from build123d import *

# Parameters (mm, degrees)
F0_W       = 52.5
F0_H       = 3
F1_DEPTH   = 6
F0_H_2     = 6
F2_DEPTH   = 3
F4_SIZE    = 2.99999
F5_SIZE2   = 6
F5_SIZE    = 12
F5_2_SIZE2 = 6
F5_2_SIZE  = 12
F6_W       = 4
F6_H       = 39
F7_DEPTH   = 2
F8_SIZE    = 1.99999
F10_DEPTH  = 3
F13_DEPTH  = 3
F12_W      = 4
F12_H      = 39
F15_DEPTH  = 2
F16_SIZE   = 1.99999
F17_SIZE   = 1.99999
F18_DEPTH  = 25
F19_R      = 5


# Not quite as in the source:
# - a fillet or chamfer is up to 0.001 mm smaller than in the source, because OpenCascade refuses the exact size


with BuildPart() as f1:
    # F0 (on Top) → F1 (new body)
    with BuildSketch(Plane.XY):
        with Locations((0, 27)):
            Rectangle(F0_W, F0_H)
        with Locations((0, 24)):
            Rectangle(F0_W, F0_H)
    extrude(amount=F1_DEPTH)


with BuildPart() as f1b:
    # F0 (on Top) → F1, piece 2 (new body)
    with BuildSketch(Plane.XY):
        Rectangle(F0_W, F0_H_2)
    extrude(amount=F1_DEPTH)


with BuildPart() as f1c:
    # F0 (on Top) → F1, piece 3 (new body)
    with BuildSketch(Plane.XY):
        with Locations((0, -24)):
            Rectangle(F0_W, F0_H)
        with Locations((0, -27)):
            Rectangle(F0_W, F0_H)
    extrude(amount=F1_DEPTH)


with BuildPart() as f2:
    # F0 (on Top) → F2 (new body)
    with BuildSketch(Plane.XY):
        Polygon((-38.25, 28.5), (-38.25, -28.5), (-38.25, -31.5), (-35.25, -31.5), (35.25, -31.5), (38.25, -31.5), (38.25, -28.5), (38.25, 28.5), (38.25, 31.5), (35.25, 31.5), (-35.25, 31.5), (-38.25, 31.5), align=None)
        with BuildLine():
            Line((-26.25, -25.5), (-29.75, -25.5))
            ThreePointArc((-29.75, -25.5), (-34.017766953, -27.267766953), (-32.25, -23))
            Line((-32.25, -23), (-32.25, -2.5))
            ThreePointArc((-32.25, -2.5), (-34.75, 0), (-32.25, 2.5))
            Line((-32.25, 2.5), (-32.25, 23))
            ThreePointArc((-32.25, 23), (-34.017766953, 27.267766953), (-29.75, 25.5))
            Line((-29.75, 25.5), (-26.25, 25.5))
            Line((-26.25, 25.5), (-26.25, 28.5))
            Line((-26.25, 28.5), (26.25, 28.5))
            Line((26.25, 28.5), (26.25, 25.5))
            Line((26.25, 25.5), (29.75, 25.5))
            ThreePointArc((29.75, 25.5), (32.25, 28), (34.75, 25.5))
            ThreePointArc((34.75, 25.5), (34.017766953, 23.732233047), (32.25, 23))
            Line((32.25, 23), (32.25, 2.5))
            ThreePointArc((32.25, 2.5), (34.017766953, 1.767766953), (34.75, 0))
            ThreePointArc((34.75, 0), (34.017766953, -1.767766953), (32.25, -2.5))
            Line((32.25, -2.5), (32.25, -23))
            ThreePointArc((32.25, -23), (34.017766953, -23.732233047), (34.75, -25.5))
            ThreePointArc((34.75, -25.5), (32.25, -28), (29.75, -25.5))
            Line((29.75, -25.5), (26.25, -25.5))
            Line((26.25, -25.5), (26.25, -28.5))
            Line((26.25, -28.5), (-26.25, -28.5))
            Line((-26.25, -28.5), (-26.25, -25.5))
        make_face(mode=Mode.SUBTRACT)
        with BuildLine():
            ThreePointArc((-32.25, -23), (-30.482233047, -23.732233047), (-29.75, -25.5))
            Line((-29.75, -25.5), (-26.25, -25.5))
            Line((-26.25, -25.5), (-26.25, -22.5))
            Line((-26.25, -22.5), (26.25, -22.5))
            Line((26.25, -22.5), (26.25, -25.5))
            Line((26.25, -25.5), (29.75, -25.5))
            ThreePointArc((29.75, -25.5), (30.482233047, -23.732233047), (32.25, -23))
            Line((32.25, -23), (32.25, -2.5))
            ThreePointArc((32.25, -2.5), (29.75, 0), (32.25, 2.5))
            Line((32.25, 2.5), (32.25, 23))
            ThreePointArc((32.25, 23), (30.482233047, 23.732233047), (29.75, 25.5))
            Line((29.75, 25.5), (26.25, 25.5))
            Line((26.25, 25.5), (26.25, 22.5))
            Line((26.25, 22.5), (-26.25, 22.5))
            Line((-26.25, 22.5), (-26.25, 25.5))
            Line((-26.25, 25.5), (-29.75, 25.5))
            ThreePointArc((-29.75, 25.5), (-30.482233047, 23.732233047), (-32.25, 23))
            Line((-32.25, 23), (-32.25, 2.5))
            ThreePointArc((-32.25, 2.5), (-30.482233047, 1.767766953), (-29.75, 0))
            ThreePointArc((-29.75, 0), (-30.482233047, -1.767766953), (-32.25, -2.5))
            Line((-32.25, -2.5), (-32.25, -23))
        make_face()
        with BuildLine():
            ThreePointArc((-23.25, -19.5), (-25.3713203436, -18.6213203436), (-26.25, -16.5))
            Line((-26.25, -16.5), (-26.25, -9))
            ThreePointArc((-26.25, -9), (-25.3713203436, -6.8786796564), (-23.25, -6))
            Line((-23.25, -6), (23.25, -6))
            ThreePointArc((23.25, -6), (25.3713203436, -6.8786796564), (26.25, -9))
            Line((26.25, -9), (26.25, -16.5))
            ThreePointArc((26.25, -16.5), (25.3713203436, -18.6213203436), (23.25, -19.5))
            Line((23.25, -19.5), (-23.25, -19.5))
        make_face(mode=Mode.SUBTRACT)
        Rectangle(F0_W, F0_H_2, mode=Mode.SUBTRACT)
        with BuildLine():
            Line((-23.25, 19.5), (23.25, 19.5))
            ThreePointArc((23.25, 19.5), (25.3713203436, 18.6213203436), (26.25, 16.5))
            Line((26.25, 16.5), (26.25, 9))
            ThreePointArc((26.25, 9), (25.3713203436, 6.8786796564), (23.25, 6))
            Line((23.25, 6), (-23.25, 6))
            ThreePointArc((-23.25, 6), (-25.3713203436, 6.8786796564), (-26.25, 9))
            Line((-26.25, 9), (-26.25, 16.5))
            ThreePointArc((-26.25, 16.5), (-25.3713203436, 18.6213203436), (-23.25, 19.5))
        make_face(mode=Mode.SUBTRACT)
        Polygon((-38.25, -31.5), (-38.25, -28.5), (-38.25, 28.5), (-38.25, 31.5), (-41.25, 31.5), (-44.25, 31.5), (-44.25, 28.5), (-44.25, -28.5), (-44.25, -31.5), (-41.25, -31.5), align=None)
        Polygon((38.25, -28.5), (38.25, -31.5), (41.25, -31.5), (44.25, -31.5), (44.25, -28.5), (44.25, 28.5), (44.25, 31.5), (41.25, 31.5), (38.25, 31.5), (38.25, 28.5), align=None)
    extrude(amount=F2_DEPTH)


with BuildPart() as f1c_1:
    add(f1c.part)

    # F3: union F1, F1b, F2
    add(f1.part)
    add(f1b.part)
    add(f2.part)

    # F4 (size 3 in the source; OpenCascade refuses exactly that, so slightly less here)
    f4_edges = [f1c_1.edges().sort_by_distance(p)[0] for p in [
        (26.25, 25.5, 6),
        (26.25, 0, 6),
        (26.25, -25.5, 6),
        (-26.25, 25.5, 6),
        (-26.25, 0, 6),
        (-26.25, -25.5, 6),
    ]]
    chamfer(f4_edges, length=F4_SIZE)

    # F5
    f5_edges = [f1c_1.edges().sort_by_distance(p)[0] for p in [
        (44.25, -31.5, 1.5),
        (44.25, 31.5, 1.5),
    ]]
    f5_side = f1c_1.faces().sort_by_distance((44.25, 0, 1.5))[0]
    chamfer(f5_edges, length=F5_SIZE, length2=F5_SIZE2, reference=f5_side)

    # F5#2
    f5_2_edges = [f1c_1.edges().sort_by_distance(p)[0] for p in [
        (-44.25, -31.5, 1.5),
        (-44.25, 31.5, 1.5),
    ]]
    f5_2_side = f1c_1.faces().sort_by_distance((-44.25, 0, 1.5))[0]
    chamfer(f5_2_edges, length=F5_2_SIZE, length2=F5_2_SIZE2, reference=f5_2_side)

    # F6 (on face) → F7 (join)
    with BuildSketch(Plane.XY.offset(3)):
        with Locations((-39.25, 0)):
            Rectangle(F6_W, F6_H)
        with Locations((39.25, 0)):
            Rectangle(F6_W, F6_H)
    extrude(amount=F7_DEPTH)

    # F8 (size 2 in the source; OpenCascade refuses exactly that, so slightly less here)
    f8_edges = [f1c_1.edges().sort_by_distance(p)[0] for p in [
        (-39.25, -19.5, 5),
        (-39.25, 19.5, 5),
        (39.25, 19.5, 5),
        (39.25, -19.5, 5),
    ]]
    chamfer(f8_edges, length=F8_SIZE)


with BuildPart() as f10:
    # F9 (on face) → F10 (new body)
    with BuildSketch(Plane(origin=(0, 0, 0), x_dir=(1, 0, 0), z_dir=(0, 0, -1))):
        Polygon((53.25, 31.5), (38.25, 31.5), (44.25, 19.5), (44.25, -19.5), (38.25, -31.5), (53.25, -31.5), align=None)
    extrude(amount=-F10_DEPTH)


with BuildPart() as f1c_2:
    add(f1c_1.part)

    # F11: union F10
    add(f10.part)


with BuildPart() as f13:
    # F12 (on face) → F13 (new body)
    with BuildSketch(Plane.XY.offset(3)):
        Polygon((-38.25, -31.5), (-44.25, -19.5), (-39.25, -31.5), align=None)
    extrude(amount=-F13_DEPTH)


with BuildPart() as f13b:
    # F12 (on face) → F13, piece 2 (new body)
    with BuildSketch(Plane.XY.offset(3)):
        Polygon((-38.25, 31.5), (-39.25, 31.5), (-44.25, 19.5), align=None)
    extrude(amount=-F13_DEPTH)


with BuildPart() as f1c_3:
    add(f1c_2.part)

    # F14: union F13b, F13
    add(f13b.part)
    add(f13.part)

    # F12 (on face) → F15 (join)
    with BuildSketch(Plane.XY.offset(3)):
        with Locations((47.25, 0)):
            Rectangle(F12_W, F12_H)
    extrude(amount=F15_DEPTH)

    # F16 (size 2 in the source; OpenCascade refuses exactly that, so slightly less here)
    f16_edges = [f1c_3.edges().sort_by_distance(p)[0] for p in [
        (47.25, -19.5, 5),
    ]]
    chamfer(f16_edges, length=F16_SIZE)

    # F17 (size 2 in the source; OpenCascade refuses exactly that, so slightly less here)
    f17_edges = [f1c_3.edges().sort_by_distance(p)[0] for p in [
        (47.25, 19.5, 5),
    ]]
    chamfer(f17_edges, length=F17_SIZE)

    # F12 (on face) → F18 (cut)
    with BuildSketch(Plane.XY.offset(3)):
        Polygon((53.25, 31.5), (39.25, 31.5), (53.25, 19.5), align=None)
        Polygon((53.25, -19.5), (39.25, -31.5), (53.25, -31.5), align=None)
    extrude(amount=-F18_DEPTH, mode=Mode.SUBTRACT)

    # F19
    f19_edges = [f1c_3.edges().sort_by_distance(p)[0] for p in [
        (39.25, -31.5, 1.5),
        (53.25, -19.5, 1.5),
        (-39.25, -31.5, 1.5),
        (-44.25, -19.5, 1.5),
        (-44.25, 19.5, 1.5),
        (-39.25, 31.5, 1.5),
        (39.25, 31.5, 1.5),
        (53.25, 19.5, 1.5),
    ]]
    fillet(f19_edges, radius=F19_R)


solid = f1c_3.part
Could you check a few things on this model? Use its own coordinates, in mm. A direction names the side the tool comes from. Round coordinates to 2 decimals unless told otherwise and drop trailing zeros. Write each loop counter-clockwise with the first axis right and the second up, starting at its lowest first coordinate (ties: lowest second). Pieces come first, ordered by that corner, then holes. Notation, with made-up numbers: (77.5, 60) - (128.5, 60) arc R17 ccw to (128.5, 88) - close; hole circle Ø9 at (8.25, 58). An arc over 180 degrees is marked (long way). Use a Markdown table: item, result.
Q1. Please list where these lines run through material, in increasing order: L1, parallel to X at y = 9, z = 4.6; L2, parallel to Y at x = -32.25, z = 0.75; L3, parallel to Y at x = 5.5, z = 0.45.
Output values:
| item | result |
|---|---|
| L1 | -41.25 to -37.25, 37.25 to 41.25, 45.25 to 49.25 |
| L2 | -31.5 to -28, -23 to -2.5, 2.5 to 23, 28 to 31.5 |
| L3 | -31.5 to -19.5, -6 to 6, 19.5 to 31.5 |
Q2. I want a section at A-A (y = -12.5). List the corners of the cut face in (x, z) for me.
Output values:
| item | result |
|---|---|
| outline | (-44.25, 0) - (-26.25, 0) - (-26.25, 3) - (-37.25, 3) - (-37.25, 5) - (-41.25, 5) - (-41.25, 3) - (-44.25, 3) - close; (26.25, 0) - (53.25, 0) - (53.25, 3) - (49.25, 3) - (49.25, 5) - (45.25, 5) - (45.25, 3) - (41.25, 3) - (41.25, 5) - (37.25, 5) - (37.25, 3) - (26.25, 3) - close |
Q3. I want a section at C-C (z = 2). Count the separate pieces of the cut face and the enclosed holes in it, plus the area to 3 significant figures.
Output values:
| item | result |
|---|---|
| separate pieces | 1 |
| enclosed holes | 8 |
| area | 4,390 mm2 |
Q4. For faces 1 (the flat face through (26.25, -13, 1)), 2 (the flat face through (-37.25, 0, 4)), 3 (the flat face through (-41.25, 0, 4)), 4 (the flat face through (4, -21, 3)), which set-ups out of +Z, -Z, +X, -X, +Y, -Y let a thin tool reach every point of the face, with its end or its side?
Output values:
| item | result |
|---|---|
| face 1 | +Z, -Z |
| face 2 | +Z, +Y, -Y |
| face 3 | +Z, -X, +Y, -Y |
| face 4 | +Z |
Q5. For pin 1 (0.9 mm diameter, centred on x = 6, z = 5, fed in from -Y); pin 2 (2 mm diameter, centred on x = -40, y = 5.5, fed in from +Z), each with a flat end and sliding along its axis, tell me the tip position at first contact or that it passes through.
Output values:
| item | result |
|---|---|
| pin 1 | y = -28.5 |
| pin 2 | z = 5 |
Q6. I want a section at B-B (x = 21). List the corners of the cut face in (y, z) for me.
Output values:
| item | result |
|---|---|
| outline | (-31.5, 0) - (-19.5, 0) - (-19.5, 3) - (-22.5, 3) - (-22.5, 6) - (-28.5, 6) - (-28.5, 3) - (-31.5, 3) - close; (-6, 0) - (6, 0) - (6, 3) - (3, 3) - (3, 6) - (-3, 6) - (-3, 3) - (-6, 3) - close; (19.5, 0) - (31.5, 0) - (31.5, 3) - (28.5, 3) - (28.5, 6) - (22.5, 6) - (22.5, 3) - (19.5, 3) - close |
Q7. I want a section at D-D (x = -28). List the corners of the cut face in (y, z) for me, plus the area to 3 significant figures.
Output values:
| item | result |
|---|---|
| outline | (-31.5, 0) - (31.5, 0) - (31.5, 3) - (-31.5, 3) - close |
| area | 189 mm2 |
